Design review of the part built by this model. Coordinates are the model's own, in mm. Coordinates: 2 decimals unless noted, no trailing zeros. Loops run counter-clockwise (first coordinate to the right, second up) from the corner with the lowest first, then second, coordinate; pieces in that order, holes last.
Q1. Add section B-B on y = 39. Give the number of separate pieces and of enclosed holes in the cut face, and give its area (3 significant figures).
Q2. For P1, Ø2, axis at y = 38, z = 4.5, coming from the +X side, flat-tipped, find the tip position at first contact; note if it passes through.
Q3. Add section A-A on z = 1.85. Give the boundary of the cut face in (x, y), and give its area (3 significant figures).
Q4. Add section C-C on y = 88. Give the boundary of the cut face in (x, z).
Q5. Wall thickness on probe 1 along Y at (x, z) = (28, 0.4); probe 2 along X at (y, z) = (30, 1.3); probe 3 along X at (y, z) = (17.5, 0.35): over which ranges is each line inside the solid? List them lowest first.
```python
from build123d import *

# Parameters (mm, degrees)
F0_R     = 17.5846989279
F1_DEPTH = 5
F2_R     = 15
F3_SIZE  = 1


# Not quite as in the source:
# - a feature names something its author has since deleted; it is built from what else it names


with BuildPart() as f1:
    # F0 (on Top) → F1 (new body)
    with BuildSketch(Plane.XY):
        Polygon((0, 127), (0, 0), (127, 0), align=None)
        with Locations((24.1695605218, 24.1695605218)):
            Circle(F0_R, mode=Mode.SUBTRACT)
        with Locations((67.0569464564, 24.1695605218)):
            Circle(F0_R, mode=Mode.SUBTRACT)
        with Locations((24.1695605218, 67.0569464564)):
            Circle(F0_R, mode=Mode.SUBTRACT)
    extrude(amount=F1_DEPTH)

    # F2
    f2_edges = [f1.edges().sort_by_distance(p)[0] for p in [
        (127, 0, 2.5),
        (0, 0, 2.5),
        (0, 127, 2.5),
    ]]
    fillet(f2_edges, radius=F2_R)

    # F3
    f3_edges = [f1.edges().sort_by_distance(p)[0] for p in [
        (104.64499, 9.259749, 5),
        (63.5, 63.5, 0),
        (6.584862, 24.169561, 5),
        (49.472248, 24.169561, 5),
        (6.584862, 67.056946, 0),
        (6.584862, 24.169561, 0),
        (49.472248, 24.169561, 0),
        (6.584862, 67.056946, 5),
        (0, 52.893398, 0),
        (0, 52.893398, 5),
        (9.259749, 104.64499, 0),
        (4.393398, 4.393398, 0),
        (52.893398, 0, 0),
        (104.64499, 9.259749, 0),
        (9.259749, 104.64499, 5),
        (4.393398, 4.393398, 5),
        (63.5, 63.5, 5),
        (52.893398, 0, 5),
    ]]
    chamfer(f3_edges, length=F3_SIZE)


solid = f1.part
```
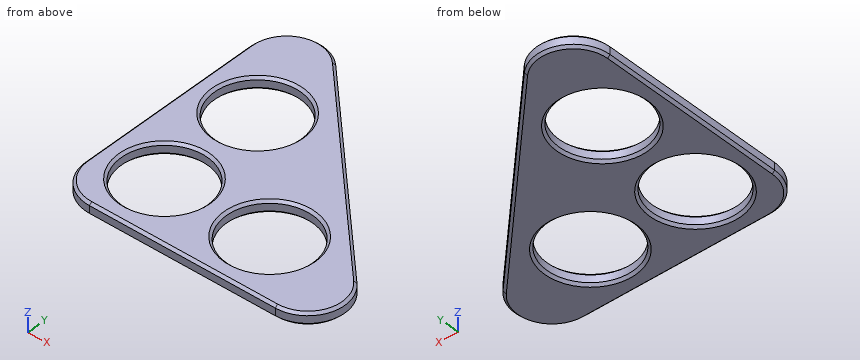
Entries:
1. separate pieces: 3
1. enclosed holes: 0
1. area: 241 mm2
2. P1: stops at x = 89.87
3. outline: (0, 15) arc R15 ccw to (15, 0) - (90.79, 0) arc R15 ccw to (101.39, 25.61) - (25.61, 101.39) arc R15 ccw to (0, 90.79) - close; hole circle Ø35.17 at (24.17, 24.17); hole circle Ø35.17 at (24.17, 67.06); hole circle Ø35.17 at (67.06, 24.17)
3. area: 4,550 mm2
4. outline: (0, 1) - (1, 0) - (37.59, 0) - (39, 1) - (39, 4) - (37.59, 5) - (1, 5) - (0, 4) - close
5. probe 1: y = 0.6 to 6.39, 41.95 to 49.28, 84.83 to 98.15
5. probe 2: x = 0 to 7.58, 40.76 to 50.47, 83.65 to 97
5. probe 3: x = 0.65 to 7.2, 41.14 to 50.09, 84.03 to 104.92
